```python
from build123d import *

# Parameters (mm, degrees)
EXTRUDE_1_DEPTH          = 85
SKETCH_3_R               = 2.2499999999999964
SKETCH_3_R_2             = 2.2500000000000018
CUT_EXTRUDE_1_DEPTH      = 19.999999999999996
EXTRUDE_2_DEPTH          = 3
EXTRUDE_3_DEPTH          = 3
FILLET_1_R               = 5
SKETCH_6_R               = 1.6999999999999973
SKETCH_6_R_2             = 1.7000000000000015
SKETCH_6_R_3             = 1.6999999999999984
SKETCH_6_R_4             = 1.6999999999999995
CUT_EXTRUDE_2_DEPTH      = 10
CUT_EXTRUDE_3_DEPTH      = 185.8550415825309
CUT_EXTRUDE_3_DEPTH_BACK = 185.8550415825309
SKETCH_8_W               = 29.999999999999993
SKETCH_8_H               = 12
SKETCH_8_H_2             = 12.000000000000002
CUT_EXTRUDE_4_DEPTH      = 150
EXTRUDE_4_DEPTH          = 5
FILLET_4_R               = 3
FILLET_5_R               = 10
FILLET_6_R               = 10


with BuildPart() as part:
    # 草图2 → 凸台-拉伸1 (new body)
    with BuildSketch(Plane.XY):
        Polygon((0, 0), (-31.18675362266453, 146.7221401100707), (-36.07749162633355, 145.6825816559819), (-6.174485782675303, 5), (-70, 4.999999999999992), (-70, 0), align=None)
    extrude(amount=EXTRUDE_1_DEPTH)

    # 草图3 → 切除-拉伸1 (cut)
    with BuildSketch(Plane(origin=(0, 0, 0), x_dir=(0, 0, -1), z_dir=(0.9781476007338048, 0.20791169081776356, 0))):
        with Locations(Location((-79.99999999999997, 79.99999999999996, 0), (0, 0, 90))):
            Circle(SKETCH_3_R)
        with Locations(Location((-4.999999999999984, 79.99999999999996, 0), (0, 0, 90))):
            Circle(SKETCH_3_R_2)
    extrude(amount=-CUT_EXTRUDE_1_DEPTH, mode=Mode.SUBTRACT)

    # 草图4 → 凸台-拉伸2 (add)
    with BuildSketch(Plane.XY.offset(85)):
        Polygon((-36.07749162633355, 145.6825816559819), (-70, 4.999999999999992), (-70, 0), (0, 0), (-31.18675362266453, 146.7221401100707), align=None)
    extrude(amount=EXTRUDE_2_DEPTH)

    # 草图5 → 凸台-拉伸3 (add)
    with BuildSketch(Plane(origin=(0, 0, 0), x_dir=(-1, 0, 0), z_dir=(0, 0, -1))):
        Polygon((36.07749162633355, 145.6825816559819), (31.18675362266453, 146.7221401100707), (0, 0), (70, 0), (70, 4.999999999999992), align=None)
    extrude(amount=EXTRUDE_3_DEPTH)

    # 圆角1
    fillet_1_edges = [part.edges().sort_by_distance(p)[0] for p in [
        (0, 0, 42.5),
    ]]
    fillet(fillet_1_edges, radius=FILLET_1_R)

    # 草图6 → 切除-拉伸2 (cut)
    with BuildSketch(Plane.XZ):
        with Locations(Location((-65, 67.5, 0), (0, 0, 270))):
            Circle(SKETCH_6_R)
        with Locations(Location((-34.99999999999999, 67.5, 0), (0, 0, 270))):
            Circle(SKETCH_6_R_2)
        with Locations(Location((-65.00000000000001, 17.5, 0), (0, 0, 270))):
            Circle(SKETCH_6_R_3)
        with Locations(Location((-34.999999999999986, 17.5, 0), (0, 0, 270))):
            Circle(SKETCH_6_R_4)
    extrude(amount=-CUT_EXTRUDE_2_DEPTH, mode=Mode.SUBTRACT)

    # 草图7 → 切除-拉伸3 (cut, two sides: drawn at the far end of the back side and taken through both)
    with BuildSketch(Plane.XY.offset(-CUT_EXTRUDE_3_DEPTH_BACK)):
        Polygon((-36.07749162633355, 145.6825816559819), (-16.94740107603117, 55.68258165598189), (-57.7790108740802, 55.682581655981885), align=None)
    extrude(amount=CUT_EXTRUDE_3_DEPTH + CUT_EXTRUDE_3_DEPTH_BACK, mode=Mode.SUBTRACT)

    # 草图8 → 切除-拉伸4 (cut)
    with BuildSketch(Plane.XZ):
        with Locations((-55, 82.00000000000001)):
            Rectangle(SKETCH_8_W, SKETCH_8_H)
        with Locations((-55, 3.000000000000001)):
            Rectangle(SKETCH_8_W, SKETCH_8_H_2)
    extrude(amount=-CUT_EXTRUDE_4_DEPTH, mode=Mode.SUBTRACT)

    # 草图9 → 凸台-拉伸4 (add)
    with BuildSketch(Plane.XY.offset(45.000000000000014)):
        Polygon((-36.077491626333554, 145.6825816559819), (-70, 5), (-6.174485782675303, 5), align=None)
    extrude(amount=-EXTRUDE_4_DEPTH)

    # 圆角4
    fillet_4_edges = [part.edges().sort_by_distance(p)[0] for p in [
        (-16.94740107603117, 55.68258165598189, -1.5),
        (-6.174485782675303, 5, 65),
        (-6.174485782675303, 5, 20.000000000000007),
        (-21.125988704504426, 75.34129082799095, 40.000000000000014),
        (-38.08724289133765, 5, 40.000000000000014),
        (-21.125988704504426, 75.34129082799095, 45.000000000000014),
        (-38.08724289133765, 5, 45.000000000000014),
        (-23.087242891337652, 4.999999999999998, 85),
        (-23.087242891337652, 4.999999999999998, 0),
        (-11.560943429353237, 30.34129082799096, 0),
        (-11.560943429353237, 30.34129082799096, 85),
        (-16.94740107603117, 55.68258165598189, 86.5),
    ]]
    fillet(fillet_4_edges, radius=FILLET_4_R)

    # 圆角5
    fillet_5_edges = [part.edges().sort_by_distance(p)[0] for p in [
        (-70, 2.499999999999996, 9.000000000000002),
        (-70, 2.499999999999996, 76.00000000000001),
        (-40.00000000000001, 2.499999999999998, 76.00000000000001),
        (-40.00000000000001, 2.499999999999998, 9.000000000000002),
    ]]
    fillet(fillet_5_edges, radius=FILLET_5_R)

    # 圆角6
    fillet_6_edges = [part.edges().sort_by_distance(p)[0] for p in [
        (-33.63212262449904, 146.2023608830263, 88),
        (-33.63212262449904, 146.2023608830263, -3),
    ]]
    fillet(fillet_6_edges, radius=FILLET_6_R)


solid = part.part
```
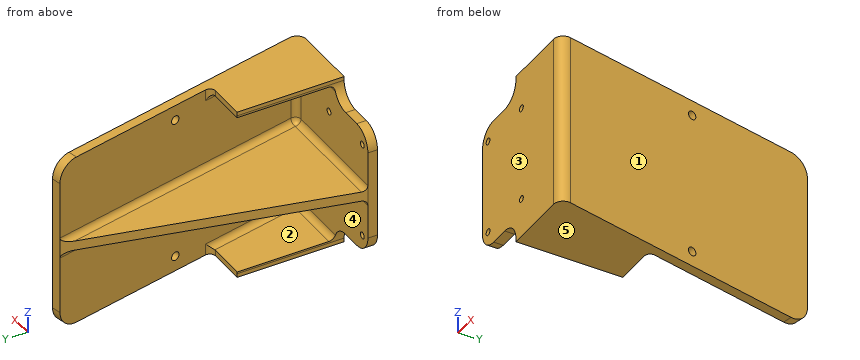
Source: CAD feature listing. Evaluate the final solid. Frame: model axes, mm. Face numbers are marked on the shaded views. A direction names the side the tool comes from. Coordinates: 2 decimals unless noted, no trailing zeros. Write each loop counter-clockwise with the first axis right and the second up, starting at its lowest first coordinate (ties: lowest second). Pieces come first, ordered by that corner, then holes. Notation, with made-up numbers: (-21, 54.5) - (17, 54.5) arc R13 ccw to (17, 67.5) - close; hole circle Ø4 at (60, -14). An arc over 180 degrees is marked (long way). Answer as a JSON object with one key per item and string values.
Q1. First-contact query: pin 1 Ø2 at (x, z) = (-65, 67.5) entering from +Y; pin 2 Ø1 at (y, z) = (30, 86.5) entering from -X; pin 3 Ø4.5 at (x, z) = (-35, 17.5) entering from +Y; pin 4 Ø2.5 at (x, y) = (-53.5, 1.5) entering from +Z. Flat tips, straight axial feed; report the tip coordinate or a pass-through.
Ans:
{"pin 1": "passes through", "pin 2": "stops at x = -40", "pin 3": "stops at y = 146.39", "pin 4": "stops at z = 76"}
Q2. Section query B-B, the plane z = 17.5. Output: boundary loops of the cut face in (x, y), plus the area to 3 significant figures.
Ans:
{"outline": "(-69.89, 0) - (-66.7, 0) - (-66.7, 5) - (-69.89, 5) - close; (-63.3, 0) - (-36.7, 0) - (-36.7, 5) - (-63.3, 5) - close; (-36.08, 145.68) - (-6.94, 8.62) arc R3 cw to (-9.88, 5) - (-33.3, 5) - (-33.3, 0) - (-6.17, 0) arc R5 ccw to (-1.28, 6.04) - (-31.19, 146.72) - close", "area": "1,030 mm2"}
Q3. Section query A-A, the plane x = -65. Output: boundary loops of the cut face in (y, z).
Ans:
{"outline": "(0, 10.34) - (5, 10.34) - (5, 15.8) - (0, 15.8) - close; (0, 19.2) - (5, 19.2) - (5, 37) arc R3 cw to (8, 40) - (25.74, 40) - (25.74, 45) - (8, 45) arc R3 cw to (5, 48) - (5, 65.8) - (0, 65.8) - close; (0, 69.2) - (5, 69.2) - (5, 74.66) - (0, 74.66) - close"}
Q4. Section query D-D, the plane x = -58. Output: boundary loops of the cut face in (y, z).
Ans:
{"outline": "(0, 9) - (5, 9) - (5, 37) arc R3 cw to (8, 40) - (54.77, 40) - (54.77, 45) - (8, 45) arc R3 cw to (5, 48) - (5, 76) - (0, 76) - close"}
Q5. Section query C-C, the plane z = 53.5. Output: boundary loops of the cut face in (x, y).
Ans:
{"outline": "(-70, 0) - (-6.17, 0) arc R5 ccw to (-1.28, 6.04) - (-31.19, 146.72) - (-36.08, 145.68) - (-6.94, 8.62) arc R3 cw to (-9.88, 5) - (-70, 5) - close"}
Q6. Material intervals for line 1 (Z direction, x = -32.5, y = 21); line 2 (Z direction, x = -65, y = 2); line 3 (X direction, y = 2, z = 17), sorted ascending. Write a range as [from, to].
Ans:
{"line 1": "z = [-3, 0], [40, 45], [85, 88]", "line 2": "z = [10.34, 15.8], [19.2, 65.8], [69.2, 74.66]", "line 3": "x = [-69.8, -66.62], [-63.38, -36.62], [-33.38, -2.17]"}
Q7. Set-up query: the marked faces 4 and 5. Return all of +Z, -Z, +X, -X, +Y, -Y with unobstructed straight access to the full face (end or side cutting, diameter ignored); none if empty.
Ans:
{"face 4": "-X", "face 5": "-Z, +X, -X, +Y, -Y"}
Q8. Draft query along Y for the marked faces 1, 2 and 3. Return one class per face: released by +Y, released by -Y, zero draft, split by the parting line, or undercut.
Ans:
{"face 1": "released by +Y", "face 2": "undercut", "face 3": "released by -Y"}
